Read the model definition and answer for the solid it produces. Units are mm, in the model's axes. A direction names the side the tool comes from. Coordinates: 2 decimals unless noted, no trailing zeros. Write each loop counter-clockwise with the first axis right and the second up, starting at its lowest first coordinate (ties: lowest second). Pieces come first, ordered by that corner, then holes.
Item 1: Section A-A (x = 10) is taken. Give the vertices of the cut face in (y, z), then the cut area to 4 significant figures.
Item 2: Section B-B (z = 7.5) is taken. Give the vertices of the cut face in (x, y), then the cut area to 3 significant figures.
Item 3: Section D-D (z = 1.75) is taken. Give the vertices of the cut face in (x, y).
Item 4: Each of these flat-tipped pins is pushed along its axis until it touches: P1, Ø6.5, axis at x = 0.5, z = 8.5, coming from the +Y side; P2, Ø7.5, axis at x = -5, z = 6, coming from the -Y side; P3, Ø4.5, axis at x = 22.5, z = 7.5, coming from the +Y side; P4, Ø3, axis at x = 30, z = 2, coming from the -Y side. Where does it stop, or does it pass through?
Item 5: Section C-C (y = -16) is taken. Give the vertices of the cut face in (x, z), then the cut area to 3 significant figures.
Item 6: Straight lines are drawn through the part: probe 1 along Y at (x, z) = (-40, 4.5); probe 2 along Z at (x, y) = (22.5, -3.25); probe 3 along X at (y, z) = (-12.5, 9.25). For each, find the intervals that lie inside material, in ascending order.
Item 7: A tool of negligible diameter and unlimited length cuts with its end or side. For faces 5 (the face through (35.064, -18.697, 7.395)), 6 (the face through (0, -1.5, 7)), 7 (the face through (50, -20, 7)), from which of +Z, -Z, +X, -X, +Y, -Y can it reach the whole face along a straight path? Write none if from no direction.
Item 8: Determine the mould class of faces 1 (the face through (10.9, -8.5, 7.4)), 2 (the face through (-24.5, -7.6, 6)), 3 (the face through (6, -8, 15)), 4 (the face through (6, -8, 0)) for opening direction Z: released by +Z, released by -Z, zero draft, split by the parting line, or undercut.
from build123d import *

# Parameters (mm, degrees)
ESBO_O1_R                = 4
ESBO_O1_R_2              = 1.75
ESBO_O1_W                = 8
ESBO_O1_H                = 3
RESSALTO_EXTRUS_O1_DEPTH = 15
ESBO_O2_R                = 2.5
CORTE_EXTRUS_O1_DEPTH    = 15


with BuildPart() as part:
    # Esboço1 → Ressalto-extrusão1 (new body)
    with BuildSketch(Plane.XY):
        with BuildLine():
            Line((-50, -10), (-50, 0))
            Line((-50, 0), (50, 0))
            Line((50, 0), (60, 0))
            Line((60, 0), (60, -20))
            Line((60, -20), (40, -20))
            ThreePointArc((40, -20), (35, -18.660254038), (31.339745962, -15))
            Line((31.339745962, -15), (-31.339745962, -15))
            ThreePointArc((-31.339745962, -15), (-42.588190451, -19.659258263), (-50, -10))
        make_face()
        with Locations((-40, -10)):
            Circle(ESBO_O1_R, mode=Mode.SUBTRACT)
        with Locations(Location((40, -10, 0), (0, 0, 180))):
            Circle(ESBO_O1_R, mode=Mode.SUBTRACT)
        with Locations((10, -10)):
            Circle(ESBO_O1_R_2, mode=Mode.SUBTRACT)
        with Locations((-10, -10)):
            Circle(ESBO_O1_R_2, mode=Mode.SUBTRACT)
        with Locations((0, -3)):
            Rectangle(ESBO_O1_W, ESBO_O1_H, mode=Mode.SUBTRACT)
    extrude(amount=RESSALTO_EXTRUS_O1_DEPTH)

    # Esboço2 → Corte-extrusão1 (cut)
    with BuildSketch(Plane.XZ.offset(15)):
        with Locations((22.5, 7.5)):
            Circle(ESBO_O2_R)
        with Locations((-22.5, 7.5)):
            Circle(ESBO_O2_R)
    extrude(amount=-CORTE_EXTRUS_O1_DEPTH, mode=Mode.SUBTRACT)


solid = part.part
Established:
1. outline: (-15, 0) - (-11.75, 0) - (-11.75, 15) - (-15, 15) - close; (-8.25, 0) - (0, 0) - (0, 15) - (-8.25, 15) - close
1. area: 172.5 mm2
2. outline: (-50, -10) arc R10 ccw to (-31.34, -15) - (-25, -15) - (-25, 0) - (-50, 0) - close; (-20, -15) - (20, -15) - (20, 0) - (-20, 0) - close; (25, -15) - (31.34, -15) arc R10 ccw to (40, -20) - (60, -20) - (60, 0) - (25, 0) - close; hole circle Ø8 at (-40, -10); hole circle Ø3.5 at (-10, -10); hole (-4, -4.5) - (4, -4.5) - (4, -1.5) - (-4, -1.5) - close; hole circle Ø3.5 at (10, -10); hole circle Ø8 at (40, -10)
2. area: 1,550 mm2
3. outline: (-50, -10) arc R10 ccw to (-31.34, -15) - (31.34, -15) arc R10 ccw to (40, -20) - (60, -20) - (60, 0) - (-50, 0) - close; hole circle Ø8 at (-40, -10); hole circle Ø3.5 at (-10, -10); hole (-4, -4.5) - (4, -4.5) - (4, -1.5) - (-4, -1.5) - close; hole circle Ø3.5 at (10, -10); hole circle Ø8 at (40, -10)
4. P1: stops at y = 0
4. P2: stops at y = -15
4. P3: passes through
4. P4: stops at y = -15.27
5. outline: (-48, 0) - (-32, 0) - (-32, 15) - (-48, 15) - close; (32, 0) - (60, 0) - (60, 15) - (32, 15) - close
5. area: 660 mm2
6. probe 1: y = -20 to -14, -6 to 0
6. probe 2: z = 0 to 5, 10 to 15
6. probe 3: x = -49.68 to -43.12, -36.88 to -24.29, -20.71 to 20.71, 24.29 to 36.88, 43.12 to 60
7. face 5: +Z, -Z, -Y
7. face 6: +Z, -Z
7. face 7: +Z, -Z, +X, -X, -Y
8. face 1: zero draft
8. face 2: undercut
8. face 3: released by +Z
8. face 4: released by -Z
